Could you check a few things on this model? Use its own coordinates, in mm. Coordinates: 2 decimals unless noted, no trailing zeros. Write each loop counter-clockwise with the first axis right and the second up, starting at its lowest first coordinate (ties: lowest second). Pieces come first, ordered by that corner, then holes.
```python
from build123d import *

# Parameters (mm, degrees)
CROQUIS1_W              = 50
CROQUIS1_H              = 30
SALIENTE_EXTRUIR1_DEPTH = 15
CROQUIS2_R              = 7.5
CORTAR_EXTRUIR1_DEPTH   = 55.313902456


with BuildPart() as part:
    # Croquis1 → Saliente-Extruir1 (new, symmetric)
    with BuildSketch(Plane.XY):
        with Locations((-64.227817577, 0)):
            Rectangle(CROQUIS1_W, CROQUIS1_H)
    extrude(amount=SALIENTE_EXTRUIR1_DEPTH, both=True)

    # Croquis2 → Cortar-Extruir1 (cut, through all)
    with BuildSketch(Plane.ZY.offset(89.227817577)):
        Circle(CROQUIS2_R)
    extrude(amount=-CORTAR_EXTRUIR1_DEPTH, mode=Mode.SUBTRACT)


solid = part.part
```
1. I want a section at C-C on x = -78.5. Please give me the cut outline in (y, z).
Verdict:
outline: (-15, -15) - (15, -15) - (15, 15) - (-15, 15) - close; hole circle Ø15 at (0, 0)
2. If we mould it in two halves opening along Y, with no side actions, what happens to faces 1 (the face through (-65, 15, 0)), 2 (the face through (-65, -15, 0)), 3 (the face through (-64.578, 0.33, -7.493)), 4 (the face through (-65, 0, 15))? For each: pulls with the +Y half, pulls with the -Y half, needs draft (parallel to the pull), parting line crosses it, or undercut.
Verdict:
face 1: pulls with the +Y half
face 2: pulls with the -Y half
face 3: undercut
face 4: needs draft
3. Please list where these lines run through material, in increasing order: line 1 along Y through (x, z) = (-62, 0); line 2 along Y through (x, z) = (-69, -4.5); line 3 along Z through (x, y) = (-76, 4.25).
Verdict:
line 1: y = -15 to -7.5, 7.5 to 15
line 2: y = -15 to -6, 6 to 15
line 3: z = -15 to -6.18, 6.18 to 15
4. I want a section at A-A on z = 0. Please give me the cut outline in (x, y).
Verdict:
outline: (-89.23, -15) - (-39.23, -15) - (-39.23, -7.5) - (-89.23, -7.5) - close; (-89.23, 7.5) - (-39.23, 7.5) - (-39.23, 15) - (-89.23, 15) - close
